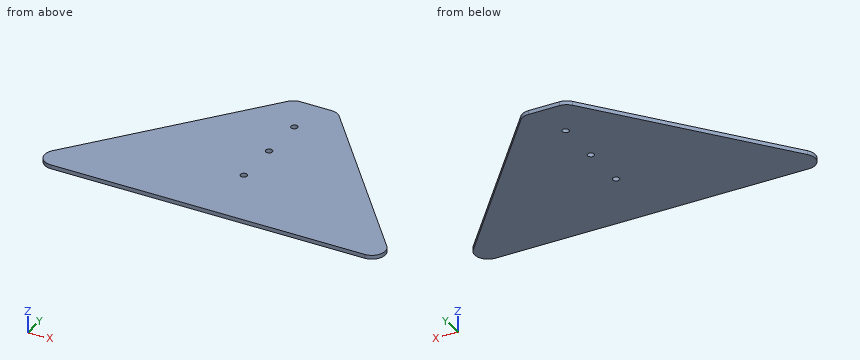
from build123d import *

# Parameters (mm, degrees)
SKETCH1_R           = 2.5
BOSS_EXTRUDE1_DEPTH = 3
FILLET1_R           = 10


with BuildPart() as part:
    # Sketch1 → Boss-Extrude1 (new body)
    with BuildSketch(Plane.XY):
        Polygon((0, 150), (-123.5, 0), (0, 0), (33, 0), (156.5, 0), (33, 150), align=None)
        with Locations((16.5, 85)):
            Circle(SKETCH1_R, mode=Mode.SUBTRACT)
        with Locations((16.5, 120)):
            Circle(SKETCH1_R, mode=Mode.SUBTRACT)
        with Locations((16.5, 50)):
            Circle(SKETCH1_R, mode=Mode.SUBTRACT)
    extrude(amount=BOSS_EXTRUDE1_DEPTH)

    # Fillet1
    fillet1_edges = [part.edges().sort_by_distance(p)[0] for p in [
        (-123.5, 0, 1.5),
        (0, 150, 1.5),
        (33, 150, 1.5),
        (156.5, 0, 1.5),
    ]]
    fillet(fillet1_edges, radius=FILLET1_R)


solid = part.part
Verification items for the finished model (mm, model axes). Coordinates: 2 decimals unless noted, no trailing zeros. Order: outer loops, then holes, each group sorted by start corner. A loop starts at its lowest first (then second) coordinate and runs counter-clockwise, first axis right, second up.
Item 1: Section check D-D, the plane y = 50. Enter the section's corners in (x, z).
Filled in:
outline: (-82.33, 0) - (14, 0) - (14, 3) - (-82.33, 3) - close; (19, 0) - (115.33, 0) - (115.33, 3) - (19, 3) - close
Item 2: Section check B-B, the plane y = 120. Enter the section's corners in (x, z), then the cut area to 3 significant figures.
Filled in:
outline: (-24.7, 0) - (14, 0) - (14, 3) - (-24.7, 3) - close; (19, 0) - (57.7, 0) - (57.7, 3) - (19, 3) - close
area: 232 mm2
Item 3: Depth check by flat-ended pin: pin 1 (6 mm diameter, centred on x = -81.5, y = 21.5, fed in from -Z). Enter the tip coordinate at first touch or a pass-through.
Filled in:
pin 1: stops at z = 0
Item 4: Section check A-A, the plane z = 1.95. Enter the section's corners in (x, y).
Filled in:
outline: (-110.03, 16.36) arc R10 ccw to (-102.31, 0) - (135.31, 0) arc R10 ccw to (143.03, 16.36) - (36, 146.36) arc R10 ccw to (28.28, 150) - (4.72, 150) arc R10 ccw to (-3, 146.36) - close; hole circle Ø5 at (16.5, 50); hole circle Ø5 at (16.5, 85); hole circle Ø5 at (16.5, 120)
Item 5: Material ranges on L1, parallel to Y at x = 16.5, z = 2.2; L2, parallel to X at y = 84.5, z = 1.8; L3, parallel to X at y = 35.5, z = 2.3, recorded low to high.
Filled in:
L1: y = 0 to 47.5, 52.5 to 82.5, 87.5 to 117.5, 122.5 to 150
L2: x = -53.93 to 14.05, 18.95 to 86.93
L3: x = -94.27 to 127.27
Item 6: Section check C-C, the plane x = 16.5. Enter the section's corners in (y, z), then the cut area to 3 significant figures.
Filled in:
outline: (0, 0) - (47.5, 0) - (47.5, 3) - (0, 3) - close; (52.5, 0) - (82.5, 0) - (82.5, 3) - (52.5, 3) - close; (87.5, 0) - (117.5, 0) - (117.5, 3) - (87.5, 3) - close; (122.5, 0) - (150, 0) - (150, 3) - (122.5, 3) - close
area: 405 mm2
